Design review of the part shown in the three views and the two pictorial views. Dimensions are in mm from the part's minimum x, y and z. Round coordinates to 2 decimals unless told otherwise and drop trailing zeros. Order: outer loops, then holes, each group sorted by start corner. A loop starts at its lowest first (then second) coordinate and runs counter-clockwise, first axis right, second up.
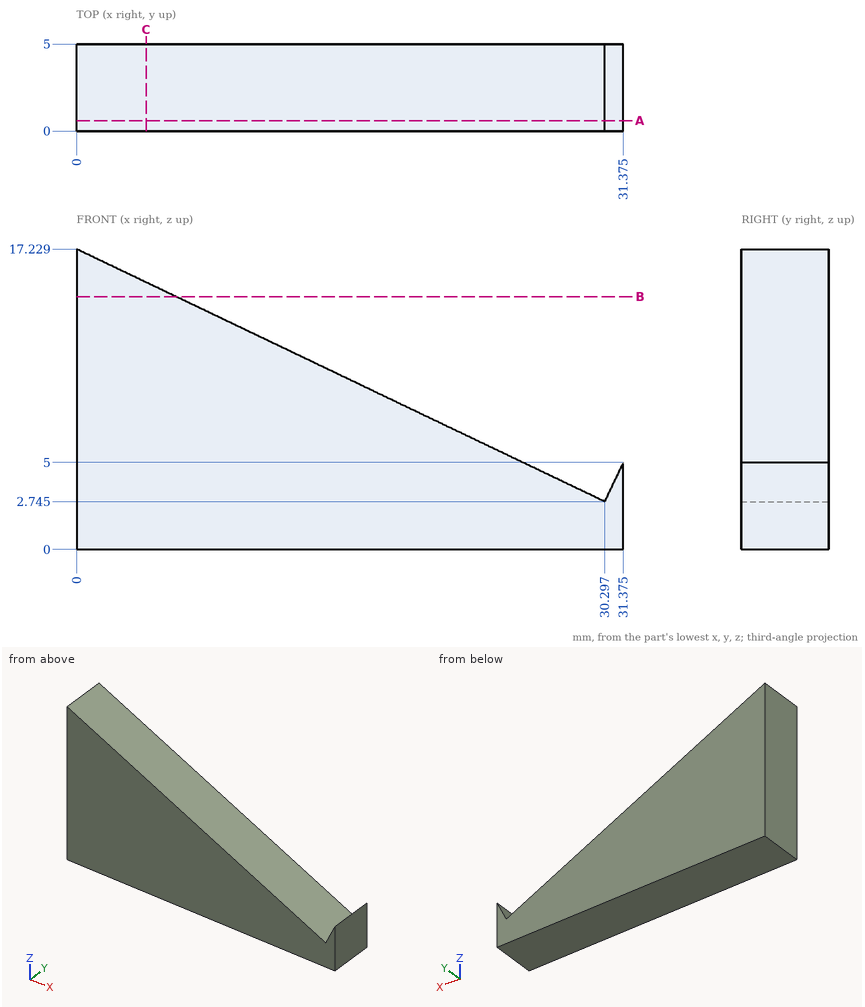
(1) To check wall thickness, follow probe 1 along X at (y, z) = (4, 4.5) (1 decimal); probe 2 along X at (y, z) = (3.7, 4) (1 decimal); probe 3 along X at (y, z) = (2.6, 7) (1 decimal). State the ranges of each line that lie inside material, in increasing order.
Data:
probe 1: x = 0 to 26.6, 31.1 to 31.4
probe 2: x = 0 to 27.7, 30.9 to 31.4
probe 3: x = 0 to 21.4
(2) Insertion check: pin 1 (2 mm diameter, centred on x = 25.5, y = 4.5, fed in from +Z) (1 decimal). The pin has a flat end and moves straight along its axis. Give the tip position at first contact, or say it passes through.
Data:
pin 1: stops at z = 5.5
(3) Consider section A-A (y = 0.6). Write out the cut boundary in (x, z) (1 decimal).
Data:
outline: (0, 0) - (31.4, 0) - (31.4, 5) - (30.3, 2.7) - (0, 17.2) - close
(4) Consider section B-B (z = 14.5). Write out the cut boundary in (x, y).
Data:
outline: (0, 0) - (5.71, 0) - (5.71, 5) - (0, 5) - close
(5) Consider section C-C (x = 4). Write out the cut boundary in (y, z).
Data:
outline: (0, 0) - (5, 0) - (5, 15.32) - (0, 15.32) - close
